Source: CAD feature listing. Evaluate the final solid. Frame: model axes, mm. Give positions to 0.01 mm unless a question says otherwise; leave off trailing zeros. Order: outer loops, then holes, each group sorted by start corner. A loop starts at its lowest first (then second) coordinate and runs counter-clockwise, first axis right, second up. Notation, with made-up numbers: M 12.25,37.5 L 36.25,37.5 A23 cw 36.25,75.5 Z; hole C 55.5,-28.75 d2. An arc over 180 degrees is marked long. Answer as a JSON object with one key per item and string values. Group by question number.
1. Section query C-C (y = 40.2). Output: boundary loops of the cut face in (x, z).
2. Section query B-B (z = 0.9). Output: boundary loops of the cut face in (x, y), plus the area to 3 significant figures.
3. Material intervals for L1, parallel to Y at x = 40.2, z = 2.8; L2, parallel to X at y = 9.8, z = 2; L3, parallel to Y at x = -52, z = 2.7, sorted ascending. Write a range as [from, to].
4. Section query A-A (x = 9.8). Output: boundary loops of the cut face in (y, z).
5. Pin query (flat end, axial travel): P1, Ø1.8, axis at x = 40.2, y = 40.2, coming from the -Z side; P2, Ø5, axis at x = 9.8, y = 40.2, coming from the +Z side. Return the tip coordinate at first contact, or that it passes through.
6. Pull-direction query (X, two-part tool) for faces 1 (the cylindrical face through (10.606, 41.465, 2.465)), 2 (the flat face through (110, 25, 2)), 3 (the cylindrical face through (99.85, 25.09, 2.46)), 4 (the flat face through (24, 50, 2)); classes: +X half, -X half, draft (parallel to the pull), parting line (faces both ways), or undercut.
7. Section query D-D (x = 102). Output: boundary loops of the cut face in (y, z), plus the area to 4 significant figures.
from build123d import *

# Parameters (mm, degrees)
ESBO_O1_W                  = 50
ESBO_O1_H                  = 50
RESSALTO_EXTRUS_O1_DEPTH   = 5
ESBO_O2_R                  = 11.5
CORTE_EXTRUS_O1_DEPTH      = 8
CORTE_EXTRUS_O1_DEPTH_BACK = 14
ESBO_O3_W                  = 60
ESBO_O3_H                  = 50
RESSALTO_EXTRUS_O2_DEPTH   = 5
ESBO_O4_R                  = 2.15
ESBO_O4_R_2                = 1.5
CORTE_EXTRUS_O2_DEPTH      = 19
CORTE_EXTRUS_O2_DEPTH_BACK = 12


with BuildPart() as part:
    # Esboço1 → Ressalto-extrusão1 (new body)
    with BuildSketch(Plane.XY):
        with Locations((25, 25)):
            Rectangle(ESBO_O1_W, ESBO_O1_H)
    extrude(amount=RESSALTO_EXTRUS_O1_DEPTH)

    # Esboço2 → Corte-extrusão1 (cut, two sides)
    with BuildSketch(Plane.XY) as corte_extrus_o1_sk:
        with Locations((25, 25)):
            Circle(ESBO_O2_R)
    extrude(amount=CORTE_EXTRUS_O1_DEPTH, mode=Mode.SUBTRACT)
    extrude(corte_extrus_o1_sk.sketch, amount=-CORTE_EXTRUS_O1_DEPTH_BACK, mode=Mode.SUBTRACT)

    # Esboço3 → Ressalto-extrusão2 (add)
    with BuildSketch(Plane.XY):
        with Locations((-30, 25)):
            Rectangle(ESBO_O3_W, ESBO_O3_H)
        with Locations((80, 25)):
            Rectangle(ESBO_O3_W, ESBO_O3_H)
    extrude(amount=RESSALTO_EXTRUS_O2_DEPTH)

    # Esboço4 → Corte-extrusão2 (cut, two sides)
    with BuildSketch(Plane.XY) as corte_extrus_o2_sk:
        with Locations((-52, 25)):
            Circle(ESBO_O4_R)
        with Locations((102, 25)):
            Circle(ESBO_O4_R)
        with Locations((9.8, 40.2)):
            Circle(ESBO_O4_R_2)
        with Locations((40.2, 40.2)):
            Circle(ESBO_O4_R_2)
        with Locations((40.2, 9.8)):
            Circle(ESBO_O4_R_2)
        with Locations((9.8, 9.8)):
            Circle(ESBO_O4_R_2)
    extrude(amount=CORTE_EXTRUS_O2_DEPTH, mode=Mode.SUBTRACT)
    extrude(corte_extrus_o2_sk.sketch, amount=-CORTE_EXTRUS_O2_DEPTH_BACK, mode=Mode.SUBTRACT)


solid = part.part
Answer sheet:
{
 "1": {"outline": "M -60,0 L 8.3,0 L 8.3,5 L -60,5 Z; M 11.3,0 L 38.7,0 L 38.7,5 L 11.3,5 Z; M 41.7,0 L 110,0 L 110,5 L 41.7,5 Z"},
 "2": {"outline": "M -60,0 L 110,0 L 110,50 L -60,50 Z; hole C -52,25 d4.3; hole C 9.8,9.8 d3; hole C 9.8,40.2 d3; hole C 25,25 d23; hole C 40.2,9.8 d3; hole C 40.2,40.2 d3; hole C 102,25 d4.3", "area": "8,030 mm^2"},
 "3": {"L1": "[0, 8.3], [11.3, 38.7], [41.7, 50]", "L2": "[-60, 8.3], [11.3, 38.7], [41.7, 110]", "L3": "[0, 22.85], [27.15, 50]"},
 "4": {"outline": "M 0,0 L 8.3,0 L 8.3,5 L 0,5 Z; M 11.3,0 L 38.7,0 L 38.7,5 L 11.3,5 Z; M 41.7,0 L 50,0 L 50,5 L 41.7,5 Z"},
 "5": {"P1": "through", "P2": "z = 5"},
 "6": {"face 1": "undercut", "face 2": "+X half", "face 3": "undercut", "face 4": "draft"},
 "7": {"outline": "M 0,0 L 22.85,0 L 22.85,5 L 0,5 Z; M 27.15,0 L 50,0 L 50,5 L 27.15,5 Z", "area": "228.5 mm^2"}
}
